Design review of the part built by this model. Coordinates are the model's own, in mm. Face numbers are marked on the shaded views. A direction names the side the tool comes from. Give positions to 0.01 mm unless a question says otherwise; leave off trailing zeros. Loops run counter-clockwise (first coordinate to the right, second up) from the corner with the lowest first, then second, coordinate; pieces in that order, holes last. Notation, with made-up numbers: (8.25, -20.75) -> (19.25, -20.75) arc R15 cw to (19.25, 6.25) -> close; hole circle Ø4 at (18.5, 61.5). An arc over 180 degrees is marked (long way). Answer as CSV lines item,"result".
from build123d import *

# Parameters (mm, degrees)
F1_DEPTH = 3
F3_DEPTH = 25


with BuildPart() as f1:
    # F0 (on Top) → F1 (new body)
    with BuildSketch(Plane.XY):
        Polygon((15, -8.660254), (15, 8.660254), (0, 17.320508), (-15, 8.660254), (-15, -8.660254), (0, -17.320508), align=None)
    extrude(amount=F1_DEPTH)

    # F2 (on face) → F3 (cut)
    with BuildSketch(Plane.XY.offset(3)):
        Polygon((0, -13.625466), (11.8, -6.812733), (11.8, 6.812733), (0, 13.625466), (-11.8, 6.812733), (-11.8, -6.812733), align=None)
    extrude(amount=-F3_DEPTH, mode=Mode.SUBTRACT)


solid = f1.part
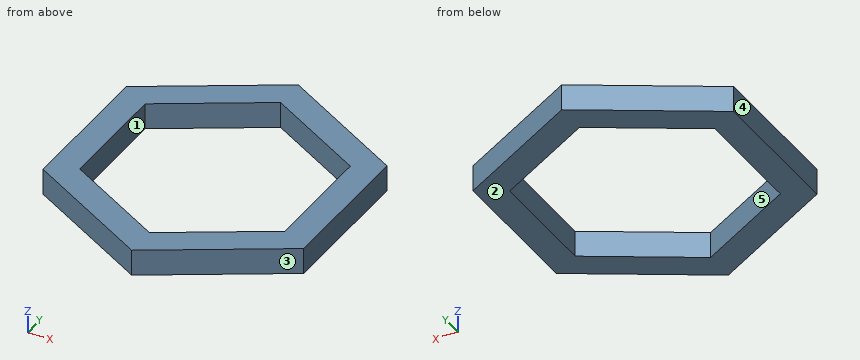
Q1. The part is to be moulded in two halves that separate along X. For the marked faces 1, 2 and 3, say which applies: pulls with the +X half, pulls with the -X half, needs draft (parallel to the pull), parting line crosses it, or undercut.
Filled sheet:
face 1,"undercut"
face 2,"needs draft"
face 3,"pulls with the +X half"
Q2. For the marked faces 4 and 5, list the 3-axis set-ups (+Z, -Z, +X, -X, +Y, -Y) from which the entire face can be reached by the end or side of a thin tool; tool diameter is ignored.
Filled sheet:
face 4,"+Z, -Z, -X, +Y, -Y"
face 5,"+Z, -Z"
Q3. We need section C-C, the plane x = -4.5. State the section outline as (y, z) points, and give its area (3 significant figures).
Filled sheet:
outline,"(-14.72, 0) -> (-11.03, 0) -> (-11.03, 3) -> (-14.72, 3) -> close; (11.03, 0) -> (14.72, 0) -> (14.72, 3) -> (11.03, 3) -> close"
area,"22.2 mm^2"
Q4. We need section B-B, the plane z = 0.85. State the section outline as (x, y) points, and give its area (3 significant figures).
Filled sheet:
outline,"(-15, -8.66) -> (0, -17.32) -> (15, -8.66) -> (15, 8.66) -> (0, 17.32) -> (-15, 8.66) -> close; hole (-11.8, -6.81) -> (0, -13.63) -> (11.8, -6.81) -> (11.8, 6.81) -> (0, 13.63) -> (-11.8, 6.81) -> close"
area,"297 mm^2"
Q5. We need section A-A, the plane y = -3. State the section outline as (x, z) points, and give its area (3 significant figures).
Filled sheet:
outline,"(-15, 0) -> (-11.8, 0) -> (-11.8, 3) -> (-15, 3) -> close; (11.8, 0) -> (15, 0) -> (15, 3) -> (11.8, 3) -> close"
area,"19.2 mm^2"
Q6. To check wall thickness, follow probe 1 along X at (y, z) = (-6.5, 2.05); probe 2 along Y at (x, z) = (-4.5, 0.8); probe 3 along Y at (x, z) = (-11, 2.05). State the ranges of each line that lie inside material, in increasing order. Write a range as from..to.
Filled sheet:
probe 1,"x = -15..-11.8, 11.8..15"
probe 2,"y = -14.72..-11.03, 11.03..14.72"
probe 3,"y = -10.97..-7.27, 7.27..10.97"
Q7. Clearance check with flat-ended pins moving along their axes: pin 1 Ø10 at (x, y) = (0.5, 5.5) entering from +Z; pin 2 Ø1.5 at (x, z) = (12, 1) entering from -Y. State where each tip first meets the part, or that it passes through.
Filled sheet:
pin 1,"passes through"
pin 2,"stops at y = -10.83"
